Work out the finished part from the listing and answer in its coordinate system (mm). A direction names the side the tool comes from. Round coordinates to 2 decimals unless told otherwise and drop trailing zeros. Order: outer loops, then holes, each group sorted by start corner. A loop starts at its lowest first (then second) coordinate and runs counter-clockwise, first axis right, second up. Notation, with made-up numbers: (5, 48) - (36, 48) arc R18 cw to (36, 52) - close; hole circle Ø8 at (54, -24.5). An arc over 180 degrees is marked (long way). Use one line per item in the form item = value. Start each with the question number.
Q1. The part is cut by section A-A on y = 15. Determine the outline of the cut face in (x, z), plus the area to 3 significant figures.
Q2. Find the intervals of material crossed by line 1 (Z direction, x = -4.25, y = 15); line 2 (Z direction, x = -0.25, y = 14); line 3 (Y direction, x = -2.5, z = 6.75), in increasing order. Write a range as [from, to].
Q3. Given P1, Ø4, axis at y = 15, z = -6.5, coming from the +X side; P2, Ø1.5, axis at y = 14.5, z = 7, coming from the -X side; P3, Ø12, axis at x = 3.5, z = 7.5, coming from the -Y side, each flat-ended and moving along its own axis, determine where each tip first touches the part or whether it passes through.
Q4. Which of the six approach directions +Z, -Z, +X, -X, +Y, -Y give full straight-line access (tool end or side, diameter ignored) to faces 1 (the cylindrical face through (13.93, -0.54, -2.44)), 2 (the cylindrical face through (-4.07, 16.5, 6.57)), 3 (the cylindrical face through (0.13, -6.07, -8.5))?
Q5. The part is cut by section D-D on y = 0. Determine the outline of the cut face in (x, z).
Q6. For a pull along Z with two mould halves and no side action, classify faces 4 (the cylindrical face through (-0.13, -6.07, 8.5)), 5 (the flat face through (-9, 21, 0)), 6 (the flat face through (1, 15, -6)), 7 (the cylindrical face through (-4.07, 16.63, -6.43)) as +Z half, -Z half, draft (parallel to the pull), parting line (faces both ways), or undercut.
Q7. The part is cut by section B-B on x = -2. Determine the outline of the cut face in (y, z).
Q8. The part is cut by section C-C on z = 0. Determine the outline of the cut face in (x, y).
from build123d import *

# Parameters (mm, degrees)
F0_W     = 57.5
F0_H     = 20
F0_R     = 2.5
F1_DEPTH = 9
F2_R     = 5
F3_R     = 2.5
F4_DEPTH = 10
F5_R     = 1.5
F5_R_2   = 1.631437
F6_DEPTH = 10


with BuildPart() as f1:
    # F0 (on Right) → F1 (new body, symmetric)
    with BuildSketch(Plane.YZ):
        with Locations((21.25, 0)):
            Rectangle(F0_W, F0_H)
        Circle(F0_R, mode=Mode.SUBTRACT)
        Circle(F0_R)
    extrude(amount=F1_DEPTH, both=True)

    # F2
    f2_edges = [f1.edges().sort_by_distance(p)[0] for p in [
        (0, -7.5, 10),
        (0, -7.5, -10),
    ]]
    fillet(f2_edges, radius=F2_R)

    # F3 (on face) → F4 (join)
    with BuildSketch(Plane.YZ.offset(9)):
        Circle(F3_R)
    extrude(amount=F4_DEPTH)

    # F5 (on face) → F6 (cut)
    with BuildSketch(Plane(origin=(-9, 0, 0), x_dir=(0, -1, 0), z_dir=(-1, 0, 0))):
        with Locations((-15, 6.5)):
            Circle(F5_R)
        with Locations((-15, -6.5)):
            Circle(F5_R_2)
    extrude(amount=-F6_DEPTH, mode=Mode.SUBTRACT)


solid = f1.part
Found:
q1.outline = (-9, -10) - (9, -10) - (9, 10) - (-9, 10) - (-9, 8) - (1, 8) - (1, 5) - (-9, 5) - (-9, -4.87) - (1, -4.87) - (1, -8.13) - (-9, -8.13) - close
q1.area = 297 mm²
q2.line_1 = [-10, -8.13], [-4.87, 5], [8, 10]
q2.line_2 = [-10, -7.79], [-5.21, 5.38], [7.62, 10]
q2.line_3 = [-7.18, 13.52], [16.48, 50]
q3.P1 = 9
q3.P2 = 1
q3.P3 = -7.5
q4.face_1 = +X
q4.face_2 = -X
q4.face_3 = -Z, +X, -X, -Y
q5.outline = (-9, -10) - (9, -10) - (9, -2.5) - (19, -2.5) - (19, 2.5) - (9, 2.5) - (9, 10) - (-9, 10) - close
q6.face_4 = +Z half
q6.face_5 = draft
q6.face_6 = undercut
q6.face_7 = undercut
q7.outline = (-7.5, -5) arc R5 ccw to (-2.5, -10) - (50, -10) - (50, 10) - (-2.5, 10) arc R5 ccw to (-7.5, 5) - close; hole circle Ø3.26 at (15, -6.5); hole circle Ø3 at (15, 6.5)
q8.outline = (-9, -7.5) - (9, -7.5) - (9, -2.5) - (19, -2.5) - (19, 2.5) - (9, 2.5) - (9, 50) - (-9, 50) - close
